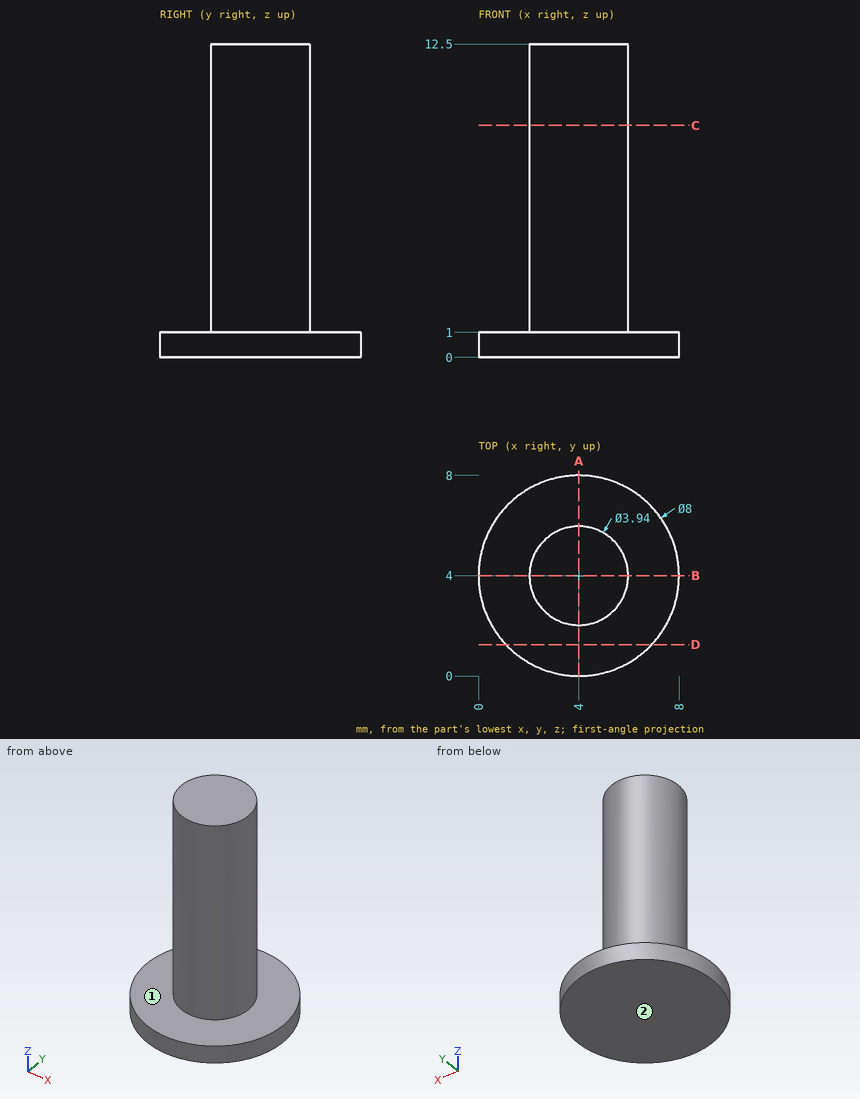
Source: three-view drawing plus pictorial views. Frame: mm from the lowest corner of the part. A direction names the side the tool comes from. Round coordinates to 2 decimals unless told otherwise and drop trailing zeros. Loops run counter-clockwise (first coordinate to the right, second up) from the corner with the lowest first, then second, coordinate; pieces in that order, holes last. Notation, with made-up numbers: M -17.5,-11 L 21.5,-11 A19 cw 21.5,0 Z; hole C 48.25,43.25 d3. An arc over 180 degrees is marked long. Answer as CSV lines item,"result".
Q1. Cut plane D-D (y = 1.25). Return the cut outline in (x, z).
Verdict:
outline,"M 1.1,0 L 6.9,0 L 6.9,1 L 1.1,1 Z"
Q2. Cut plane A-A (x = 4). Return the cut outline in (y, z).
Verdict:
outline,"M 0,0 L 8,0 L 8,1 L 5.97,1 L 5.97,12.5 L 2.03,12.5 L 2.03,1 L 0,1 Z"
Q3. Cut plane C-C (z = 9.25). Return the cut outline in (x, y), plus the area to 3 significant figures.
Verdict:
outline,"C 4,4 d3.94"
area,"12.2 mm^2"
Q4. Contact query for flat-ended pins moving along their axis: pin 1 (1 mm diameter, centred on x = 4, z = 10, fed in from +Y); pin 2 (1 mm diameter, centred on x = 5, z = 9.5, fed in from -Y); pin 3 (2 mm diameter, centred on x = 6.5, z = 8.5, fed in from +Y). Output: stop coordinate, or through.
Verdict:
pin 1,"stops at y = 5.97"
pin 2,"stops at y = 2.09"
pin 3,"stops at y = 5.28"
Q5. Line query: line 1 along Y through (x, z) = (4, 10.5); line 2 along Z through (x, y) = (5.75, 5); line 3 along X through (y, z) = (3.75, 10). Output: solid intervals per line, ascending.
Verdict:
line 1,"y = 2.03 to 5.97"
line 2,"z = 0 to 1"
line 3,"x = 2.05 to 5.95"
Q6. Reachability of the marked faces 1 and 2 from +Z, -Z, +X, -X, +Y, -Y: full face, straight path, thin tool, end or side. Return the list, or none.
Verdict:
face 1,"+Z"
face 2,"-Z, +X, -X, +Y, -Y"
